Autodesk Inventor part; units mm, degrees
ref_plane "YZ Plane" through (0, 0, 0) normal (1, 0, 0) x (0, 1, 0)
ref_plane "XZ Plane" through (0, 0, 0) normal (0, 1, 0) x (-1, 0, 0)
ref_plane "XY Plane" through (0, 0, 0) normal (0, 0, 1) x (1, 0, 0)
sketch "Sketch1" plane through (0, 0, 0) normal (0, 0, 1) x (1, 0, 0)
  line L0 (-176.5, -25) -> (176.5, -25)
  line L1 (176.5, -25) -> (176.5, 25)
  line L2 (176.5, 25) -> (-176.5, 25)
  line L3 (-176.5, 25) -> (-176.5, -25)
  line L4 (-176.5, -25) -> (176.5, 25) construction
  line L5 (176.5, -25) -> (-176.5, 25) construction
  point P0 (0, 0)
  dimension "d0" = 50
  dimension "d1" = 353
extrude "Extrusion1" add sketch "Sketch1" along normal blind 6.35
sketch "Sketch2" plane through (0, 0, 6.35) normal (0, 0, 1) x (1, 0, 0)
  line L0 (-176.5, -25) -> (176.5, -25)
  line L1 (-176.5, 25) -> (-176.5, -25)
  line L2 (0, 0) -> (0, -33.6266)
  point P0 (-147.4, -15.1)
  point P1 (147.4, -15.1)
  point P2 (-170.6, -15.1)
  point P3 (-147.4, 8.1)
  point P4 (-170.6, 8.1)
  point P5 (170.6, -15.1)
  point P6 (147.4, 8.1)
  point P7 (170.6, 8.1)
  dimension "d4" = 294.8
  dimension "d5" = 147.4
  dimension "d6" = 9.9
  dimension "d9" = 23.2
  dimension "d12" = 23.2
hole "Hole1" at (-147.4, -15.1, 6.35) at (147.4, -15.1, 6.35) at (-170.6, -15.1, 6.35) at (-147.4, 8.1, 6.35) at (-170.6, 8.1, 6.35) at (170.6, -15.1, 6.35) at (170.6, 8.1, 6.35) at (147.4, 8.1, 6.35) direction (0, 0, -1) diameter 5.4 end through all
chamfer "Chamfer1" distance 7 distance2 7.5 1 edges at (-176.5, -25, 3.175) measured on face at (-176.5, 8.3333, 2.1167)
chamfer "Chamfer2" distance 7 distance2 7.5 1 edges at (176.5, -25, 3.175) measured on face at (176.5, -8.3333, 4.2333)
sketch "Sketch3" plane through (0, 0, 6.35) normal (0, 0, 1) x (1, 0, 0)
  point P0 (0, 0)
sketch "Sketch4" plane through (0, 0, 6.35) normal (0, 0, 1) x (1, 0, 0)
  circle A0 centre (96, 14.9487) radius 1.6
  circle A1 centre (85, 10.04) radius 1.6
  circle A2 centre (74, 14.9487) radius 1.6
  circle A3 centre (-74, 14.9487) radius 1.6
  circle A4 centre (-85, 10.04) radius 1.6
  circle A5 centre (-96, 14.9487) radius 1.6
  point P0 (0, 0)
hole "Hole2" at (-96, 14.9487, 6.35) at (-85, 10.04, 6.35) at (-74, 14.9487, 6.35) at (74, 14.9487, 6.35) at (85, 10.04, 6.35) at (96, 14.9487, 6.35) direction (0, 0, -1) diameter 3.2 end through all
sketch "Sketch5" plane through (0, 0, 6.35) normal (0, 0, 1) x (1, 0, 0)
  circle A0 centre (-5, 21) radius 2.75
  circle A1 centre (-5, -5) radius 2.75
  point P0 (0, 0)
hole "Hole3" at (-5, 21, 6.35) at (-5, -5, 6.35) direction (0, 0, -1) diameter 3.2 end through all
sketch "Sketch6" plane through (0, 0, 6.35) normal (0, 0, 1) x (1, 0, 0)
  line L0 (-176.5, 9) -> (-168.109, 19)
  line L1 (-168.109, 19) -> (-118.109, 19)
  line L2 (-118.109, 19) -> (-107.7167, 25)
  line L3 (176.5, 25) -> (-176.5, 25)
  line L4 (-169, -25) -> (169, -25)
  line L5 (-139, -25) -> (-130.609, -15)
  line L6 (-130.609, -15) -> (130.609, -15)
  line L7 (130.609, -15) -> (139, -25)
  line L8 (0, 25) -> (0, 0) construction
  line L9 (-176.5, 25) -> (-176.5, -18)
  line L10 (176.5, 9) -> (168.109, 19)
  line L11 (168.109, 19) -> (118.109, 19)
  line L12 (118.109, 19) -> (107.7167, 25)
  line L13 (176.5, -18) -> (176.5, 25)
  dimension "d42" = 30
  dimension "d43" = 50
  dimension "d44" = 50
  dimension "d45" = 10
  dimension "d46" = 40
  dimension "d47" = 16
  dimension "d48" = 50
  dimension "d49" = 6
  dimension "d52" = 30
  dimension "d53" = 30
extrude "Extrusion2" cut sketch "Sketch6" against normal blind 10
fillet "Fillet1" radius 15 2 edges at (-130.609, -15, 3.175) (130.609, -15, 3.175)
fillet "Fillet1" radius 2 10 edges at (176.5, -18, 3.175) (176.5, 9, 3.175) (168.109, 19, 3.175) (118.109, 19, 3.175) (107.7167, 25, 3.175) (-118.109, 19, 3.175) (-107.7167, 25, 3.175) (-168.109, 19, 3.175) (-176.5, 9, 3.175) (-176.5, -18, 3.175)
properties part number "FRONT PLATE P1.2"
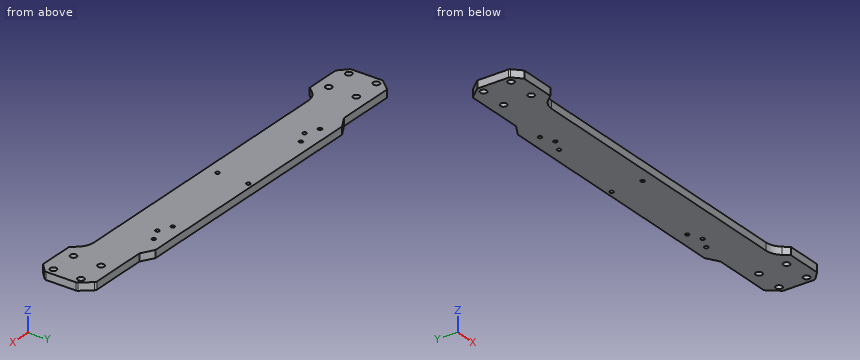
Design review of the part built by this model. Coordinates are the model's own, in mm. Coordinates: 2 decimals unless noted, no trailing zeros. Write each loop counter-clockwise with the first axis right and the second up, starting at its lowest first coordinate (ties: lowest second). Pieces come first, ordered by that corner, then holes. Notation, with made-up numbers: M -18,59.5 L 29,59.5 A31 ccw 29,84.5 Z; hole C -32.75,75 d4. An arc over 180 degrees is marked long. Answer as a JSON object with one key per item and string values.
Item 1: Add section A-A, the plane z = 2.5. State how many separate pieces and enclosed holes the cut face has, and give its area (3 significant figures).
Outcome:
{"separate pieces": "1", "enclosed holes": "16", "area": "13,800 mm²"}
Item 2: Wall thickness on probe 1 along X at (y, z) = (8, 4); probe 2 along Y at (x, z) = (-5, 2); probe 3 along Y at (x, z) = (147.4, 5): over which ranges is each line inside the solid? List them lowest first.
Outcome:
{"probe 1": "-176.5 to -173.3, -167.9 to -150.1, -144.7 to 144.7, 150.1 to 167.9, 173.3 to 176.5", "probe 2": "-15 to -6.6, -3.4 to 19.4, 22.6 to 25", "probe 3": "-25 to -17.8, -12.4 to 5.4, 10.8 to 19"}
Item 3: Add section B-B, the plane x = -27. Give the boundary of the cut face in (y, z).
Outcome:
{"outline": "M -15,0 L 25,0 L 25,6.35 L -15,6.35 Z"}
